Build history of the part. All positions in model axes, mm. Face numbers are marked on the shaded views. A direction names the side the tool comes from. Give positions to 0.01 mm unless a question says otherwise; leave off trailing zeros. Loops run counter-clockwise (first coordinate to the right, second up) from the corner with the lowest first, then second, coordinate; pieces in that order, holes last. Notation, with made-up numbers: (18.5, 64) - (44.5, 64) arc R14 ccw to (44.5, 83) - close; hole circle Ø9 at (-22.75, 12). An arc over 180 degrees is marked (long way). Return JSON: item names as keys, results as strings. Group by question number.
1) Slice it at C-C (y = 37). List the corners of the cut face in (x, z).
2) Drill centre lines: probe 1 along Z at (x, y) = (22, 6); probe 2 along Z at (x, y) = (46, 22.5); probe 3 along X at (y, z) = (26, 21). Where is each one in solid material? Low to high. Write a range as from..to.
3) Drop a flat-ended pin along its axis: pin 1 (5.5 mm diameter, centred on y = 24.5, z = 28, fed in from +X). Give the stop position or say it passes through.
4) Slice it at A-A (x = 36). List the corners of the cut face in (y, z), and give its area (3 significant figures).
5) Slice it at D-D (x = 29.5). List the corners of the cut face in (y, z).
6) Slice it at B-B (z = 35). List the corners of the cut face in (x, y).
7) Mould opens along X. For the marked faces 1, 2 and 3 say: released by +X, released by -X, zero draft, split by the parting line, or undercut.
8) 3-axis set-ups, long thin cutter, end or side, ignore diameter. For the marked faces 4, 5, 6 and 7: which of +Z, -Z, +X, -X, +Y, -Y reach the whole face in a straight line?
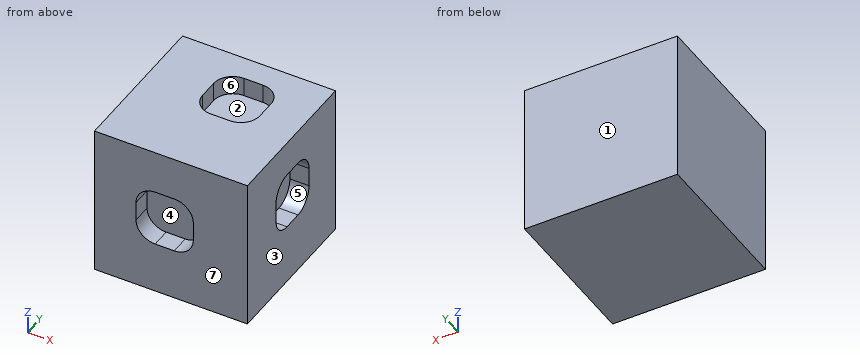
```python
from build123d import *

# Parameters (mm, degrees)
F0_W     = 50.8
F0_H     = 50.8
F1_DEPTH = 50.8
F3_DEPTH = 6.35
F5_DEPTH = 6.35
F7_DEPTH = 6.35


with BuildPart() as f1:
    # F0 (on Top) → F1 (new body)
    with BuildSketch(Plane.XY):
        with Locations((25.4, 25.4)):
            Rectangle(F0_W, F0_H)
    extrude(amount=F1_DEPTH)

    # F2 (on face) → F3 (cut)
    with BuildSketch(Plane.XY.offset(50.8)):
        with BuildLine():
            ThreePointArc((18.691622, 29.928316), (20.551494, 25.438188), (25.041622, 23.578316))
            Line((25.041622, 23.578316), (31.391622, 23.578316))
            ThreePointArc((31.391622, 23.578316), (35.88175, 25.438188), (37.741622, 29.928316))
            Line((37.741622, 29.928316), (37.741622, 36.278316))
            ThreePointArc((37.741622, 36.278316), (35.88175, 40.768444), (31.391622, 42.628316))
            Line((31.391622, 42.628316), (25.041622, 42.628316))
            ThreePointArc((25.041622, 42.628316), (20.551494, 40.768444), (18.691622, 36.278316))
            Line((18.691622, 36.278316), (18.691622, 29.928316))
        make_face()
    extrude(amount=-F3_DEPTH, mode=Mode.SUBTRACT)

    # F4 (on face) → F5 (cut)
    with BuildSketch(Plane.XZ):
        with BuildLine():
            ThreePointArc((13.781983, 23.608483), (15.641855, 19.118355), (20.131983, 17.258483))
            Line((20.131983, 17.258483), (26.481983, 17.258483))
            ThreePointArc((26.481983, 17.258483), (30.972111, 19.118355), (32.831983, 23.608483))
            Line((32.831983, 23.608483), (32.831983, 29.958483))
            ThreePointArc((32.831983, 29.958483), (30.972111, 34.448611), (26.481983, 36.308483))
            Line((26.481983, 36.308483), (20.131983, 36.308483))
            ThreePointArc((20.131983, 36.308483), (15.641855, 34.448611), (13.781983, 29.958483))
            Line((13.781983, 29.958483), (13.781983, 23.608483))
        make_face()
    extrude(amount=-F5_DEPTH, mode=Mode.SUBTRACT)

    # F6 (on face) → F7 (cut)
    with BuildSketch(Plane.YZ.offset(50.8)):
        with BuildLine():
            Line((22.827603, 20.040363), (29.177603, 20.040363))
            ThreePointArc((29.177603, 20.040363), (33.667732, 21.900235), (35.527603, 26.390363))
            Line((35.527603, 26.390363), (35.527603, 32.740363))
            ThreePointArc((35.527603, 32.740363), (33.667732, 37.230491), (29.177603, 39.090363))
            Line((29.177603, 39.090363), (22.827603, 39.090363))
            ThreePointArc((22.827603, 39.090363), (18.337475, 37.230491), (16.477603, 32.740363))
            Line((16.477603, 32.740363), (16.477603, 26.390363))
            ThreePointArc((16.477603, 26.390363), (18.337475, 21.900235), (22.827603, 20.040363))
        make_face()
    extrude(amount=-F7_DEPTH, mode=Mode.SUBTRACT)


solid = f1.part
```
Results:
{
 "1": {"outline": "(0, 0) - (50.8, 0) - (50.8, 50.8) - (37.7, 50.8) - (37.7, 44.45) - (18.73, 44.45) - (18.73, 50.8) - (0, 50.8) - close"},
 "2": {"probe 1": "0..17.26, 36.31..50.8", "probe 2": "0..20.05, 39.08..50.8", "probe 3": "0..44.45"},
 "3": {"pin 1": "x = 44.45"},
 "4": {"outline": "(0, 0) - (50.8, 0) - (50.8, 50.8) - (40.65, 50.8) - (40.65, 44.45) - (25.56, 44.45) - (25.56, 50.8) - (0, 50.8) - close", "area": "2,480 mm2"},
 "5": {"outline": "(0, 0) - (50.8, 0) - (50.8, 50.8) - (42.63, 50.8) - (42.63, 44.45) - (23.58, 44.45) - (23.58, 50.8) - (0, 50.8) - (0, 35.55) - (6.35, 35.55) - (6.35, 18.02) - (0, 18.02) - close"},
 "6": {"outline": "(0, 0) - (16.27, 0) - (16.27, 6.35) - (30.34, 6.35) - (30.34, 0) - (50.8, 0) - (50.8, 16.89) - (44.45, 16.89) - (44.45, 35.11) - (50.8, 35.11) - (50.8, 50.8) - (0, 50.8) - close"},
 "7": {"face 1": "zero draft", "face 2": "undercut", "face 3": "released by +X"},
 "8": {"face 4": "-Y", "face 5": "+X", "face 6": "+Z", "face 7": "+Z, -Z, +X, -X, -Y"}
}
